Drawing for the job (mm, zero at the part's lowest x, y, z). Give positions to 0.01 mm unless a question says otherwise; leave off trailing zeros. Order: outer loops, then holes, each group sorted by start corner. A loop starts at its lowest first (then second) coordinate and runs counter-clockwise, first axis right, second up. Notation, with made-up numbers: (66.5, -30) - (73.5, -30) arc R25 ccw to (73.5, -9) - close; hole circle Ø6 at (-40, 68.25). An arc over 180 degrees is marked (long way). One line per item, written item: value.
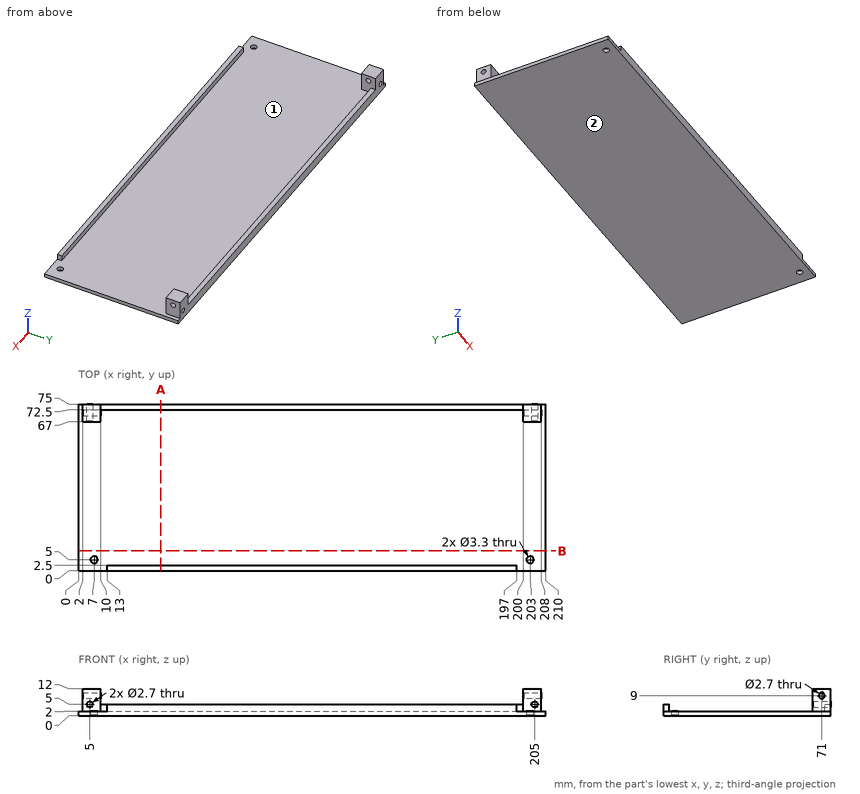
(1) Slice it at A-A, the plane x = 37. Give the cut face in (y, z).
Completed:
outline: (0, 0) - (75, 0) - (75, 5) - (72.5, 5) - (72.5, 2) - (2.5, 2) - (2.5, 5) - (0, 5) - close
(2) Slice it at B-B, the plane y = 9. Give the cut face in (x, z).
Completed:
outline: (0, 0) - (210, 0) - (210, 2) - (0, 2) - close
(3) Drill centre lines: line 1 (X direction, y = 71.75, z = 5); line 2 (Y direction, x = 155, z = 3); line 3 (Z direction, x = 168, y = 11.5). Where is each one in solid material? Low to high.
Completed:
line 1: 2 to 3.65, 6.35 to 10, 200 to 203.65, 206.35 to 208
line 2: 0 to 2.5, 72.5 to 75
line 3: 0 to 2
(4) Pin check, flat tips, straight feed: P1, Ø3.5, axis at y = 71, z = 9, coming from the +X side; P2, Ø4, axis at x = 205, z = 7.5, coming from the -Y side; P3, Ø3, axis at x = 7, y = 5, coming from the +Z side; P4, Ø1.2, axis at x = 67.5, y = 0.5, coming from the +Z side. Stop position of each tip, or through.
Completed:
P1: x = 208
P2: y = 67
P3: through
P4: z = 5
(5) Pull direction Y, two halves, no side cores. Call the marked faces 1 and 2: +Y half, -Y half, draft (parallel to the pull), parting line (faces both ways), or undercut.
Completed:
face 1: undercut
face 2: draft
